For this review, take the finished solid that the model builds, in its own axes (mm). Face numbers are marked on the shaded views. A direction names the side the tool comes from. Coordinates: 2 decimals unless noted, no trailing zeros. Write each loop counter-clockwise with the first axis right and the second up, starting at its lowest first coordinate (ties: lowest second). Pieces come first, ordered by that corner, then holes.
```python
from build123d import *

# Parameters (mm, degrees)
SKETCH1_R           = 7.5
SKETCH1_R_2         = 2.5
SKETCH1_R_3         = 2.414891735
BOSS_EXTRUDE1_DEPTH = 5


with BuildPart() as part:
    # Sketch1 → Boss-Extrude1 (new body)
    with BuildSketch(Plane.XY):
        with BuildLine():
            Line((-64.11910774, -48), (-60.619119753, -48))
            Line((-60.619119753, -48), (-60.619119753, -46))
            Line((-60.619119753, -46), (-62.119119753, -46))
            ThreePointArc((-62.119119753, -46), (-63.119119753, -45), (-62.119119753, -44))
            Line((-62.119119753, -44), (-60.619119753, -44))
            Line((-60.619119753, -44), (-60.619119753, -42))
            Line((-60.619119753, -42), (-57.619119753, -42))
            Line((-57.619119753, -42), (-57.619119753, -44))
            Line((-57.619119753, -44), (-56.119119753, -44))
            ThreePointArc((-56.119119753, -44), (-55.119119753, -45), (-56.119119753, -46))
            Line((-56.119119753, -46), (-57.619119753, -46))
            Line((-57.619119753, -46), (-57.619119753, -48))
            Line((-57.619119753, -48), (-54.119131767, -48))
            Line((-54.119131767, -48), (-54.119131767, -53))
            Line((-54.119131767, -53), (-49.119131767, -53))
            Line((-49.119131767, -53), (-49.119131767, -48.03100166))
            Line((-49.119131767, -48.03100166), (-36.926389772, -28.007003911))
            ThreePointArc((-36.926389772, -28.007003911), (-40.215260186, -13.611740859), (-54.696043275, -16.500890917))
            ThreePointArc((-54.696043275, -16.500890917), (-61.035529103, -12.290355564), (-68.334240228, -10.134780364))
            ThreePointArc((-68.334240228, -10.134780364), (-75.789232267, -11.867196487), (-79.835711336, -18.363670844))
            ThreePointArc((-79.835711336, -18.363670844), (-80.615312561, -35.401323311), (-69.11910774, -48))
            Line((-69.11910774, -48), (-69.11910774, -53))
            Line((-69.11910774, -53), (-64.11910774, -53))
            Line((-64.11910774, -53), (-64.11910774, -48))
        make_face()
        with Locations((-69.970521887, -19.999973255)):
            Circle(SKETCH1_R, mode=Mode.SUBTRACT)
        with Locations((-76.288829656, -33.523643473)):
            Circle(SKETCH1_R_2, mode=Mode.SUBTRACT)
        with Locations((-45.970521887, -22.499973255)):
            Circle(SKETCH1_R_3, mode=Mode.SUBTRACT)
    extrude(amount=BOSS_EXTRUDE1_DEPTH)


solid = part.part
```
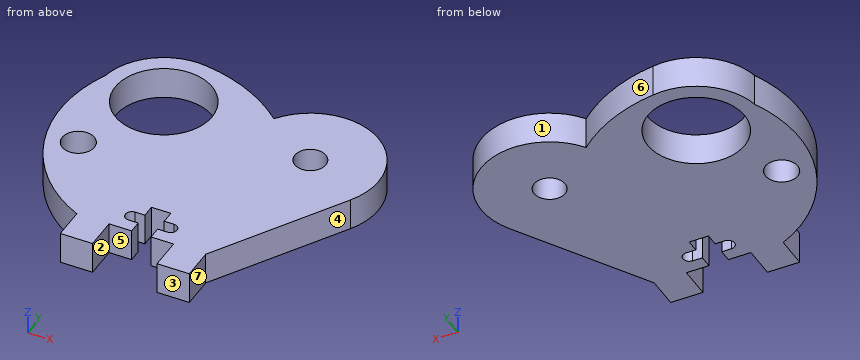
Q1. Tool access review of the marked faces 5, 6 and 7: name each direction out of +Z, -Z, +X, -X, +Y, -Y from which nothing blocks a thin tool from reaching the whole face with its end or side.
Ans:
face 5: +Z, -Z, -Y
face 6: +Z, -Z, +Y
face 7: +Z, -Z, +X, -Y
Q2. Clearance check with flat-ended pins moving along their axes: pin 1 Ø1.7 at (x, z) = (-56.5, 2.5) entering from -Y; pin 2 Ø1.5 at (x, z) = (-59.5, 2.5) entering from -Y; pin 3 Ø2.5 at (y, z) = (-50.5, 2) entering from -X. State where each tip first meets the part, or that it passes through.
Ans:
pin 1: stops at y = -48
pin 2: stops at y = -42
pin 3: stops at x = -69.12
Q3. Add section A-A (y = -26). State the section outline as (x, z) points, then the cut area to 3 significant figures.
Ans:
outline: (-81.87, 0) - (-74.47, 0) - (-74.47, 5) - (-81.87, 5) - close; (-65.47, 0) - (-35.98, 0) - (-35.98, 5) - (-65.47, 5) - close
area: 184 mm2
Q4. Add section C-C (y = -14). State the section outline as (x, z) points, then the cut area to 3 significant figures.
Ans:
outline: (-77.97, 0) - (-74.47, 0) - (-74.47, 5) - (-77.97, 5) - close; (-65.47, 0) - (-57.95, 0) - (-57.95, 5) - (-65.47, 5) - close; (-52.29, 0) - (-39.66, 0) - (-39.66, 5) - (-52.29, 5) - close
area: 118 mm2
Q5. Draft analysis for pull direction X (two halves, no side actions). For the marked faces 1, 2, 3 and 4, state which applies: +X half, -X half, draft (parallel to the pull), parting line (faces both ways), or undercut.
Ans:
face 1: undercut
face 2: undercut
face 3: draft
face 4: +X half
Q6. For probe 1 along X at (y, z) = (-14.5, 2.6); probe 2 along Y at (x, z) = (-76.5, 3.4); probe 3 along Y at (x, z) = (-76, 2.65), list the stretches that pass through material, from the lowest coordinate up.
Ans:
probe 1: x = -78.32 to -75.07, -64.87 to -57.21, -52.91 to -39.03
probe 2: y = -42.42 to -36.01, -31.03 to -23.69, -16.31 to -12.43
probe 3: y = -42.97 to -36.01, -31.04 to -24.46, -15.54 to -12.02
Q7. Add section D-D (z = 3.3). State the section outline as (x, y) points, then the cut area to 3 significant figures.
Ans:
outline: (-79.84, -18.36) arc R22.28 ccw to (-69.12, -48) - (-69.12, -53) - (-64.12, -53) - (-64.12, -48) - (-60.62, -48) - (-60.62, -46) - (-62.12, -46) arc R1 cw to (-62.12, -44) - (-60.62, -44) - (-60.62, -42) - (-57.62, -42) - (-57.62, -44) - (-56.12, -44) arc R1 cw to (-56.12, -46) - (-57.62, -46) - (-57.62, -48) - (-54.12, -48) - (-54.12, -53) - (-49.12, -53) - (-49.12, -48.03) - (-36.93, -28.01) arc R10.59 ccw to (-54.7, -16.5) arc R25.54 ccw to (-68.33, -10.13) arc R10 ccw to start; hole circle Ø5 at (-76.29, -33.52); hole circle Ø15 at (-69.97, -20); hole circle Ø4.83 at (-45.97, -22.5)
area: 1,200 mm2
Q8. Add section B-B (x = -73). State the section outline as (y, z) points, then the cut area to 3 significant figures.
Ans:
outline: (-45.67, 0) - (-26.86, 0) - (-26.86, 5) - (-45.67, 5) - close; (-13.14, 0) - (-10.47, 0) - (-10.47, 5) - (-13.14, 5) - close
area: 107 mm2
